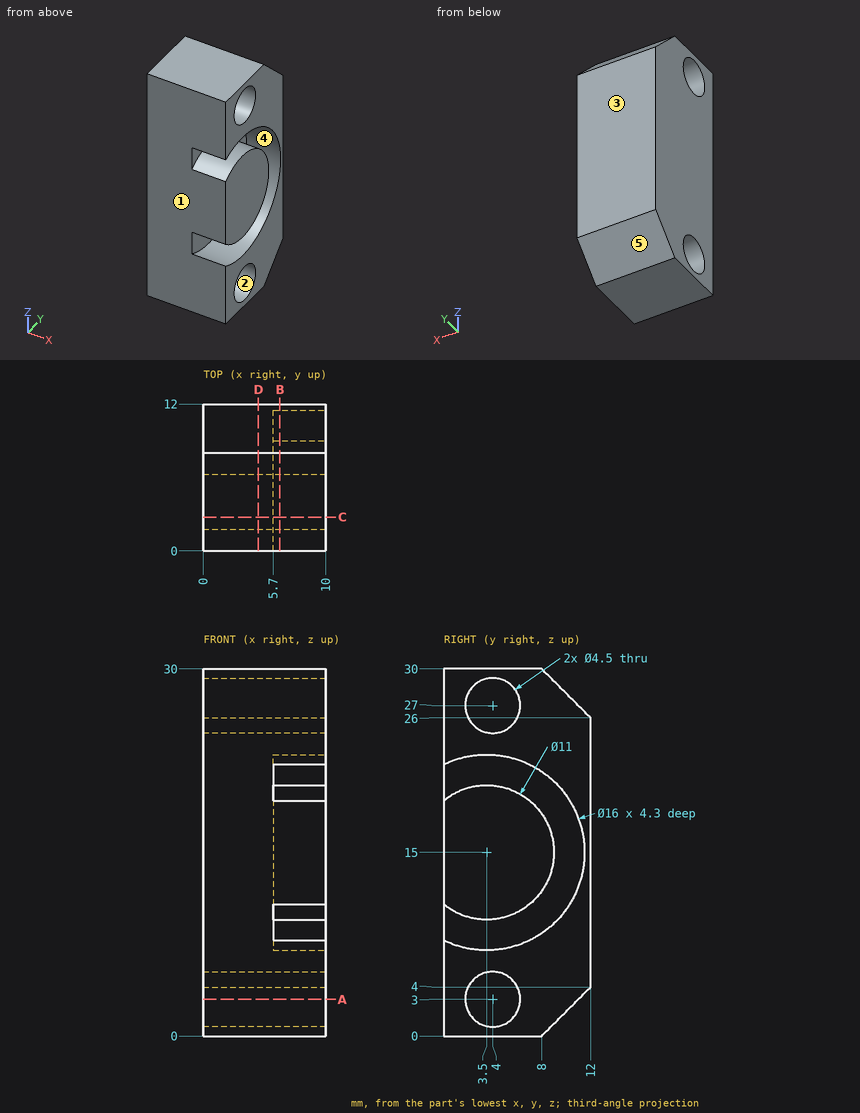
Study the drawing (mm; zero at the part's minimum x, y, z) and answer. A direction names the side the tool comes from. Coordinates: 2 decimals unless noted, no trailing zeros. Loops run counter-clockwise (first coordinate to the right, second up) from the corner with the lowest first, then second, coordinate; pieces in that order, holes last. Notation, with made-up numbers: M 17,87 L 69,87 A24 cw 69,116 Z; hole C -14,70.25 d9. An arc over 180 degrees is marked long. Answer as a JSON object with one key per item and string values. Group by question number.
Item 1: Which of the six approach directions +Z, -Z, +X, -X, +Y, -Y give full straight-line access (tool end or side, diameter ignored) to the marked faces 4 and 5?
Item 2: Determine the mould class of the marked faces 1, 2 and 3 for opening direction Y: +Y half, -Y half, draft (parallel to the pull), parting line (faces both ways), or undercut.
Item 3: Section C-C (y = 2.75) is taken. Write down the section's boundary in (x, z).
Item 4: Section D-D (x = 4.5) is taken. Write down the section's boundary in (y, z).
Item 5: Section B-B (x = 6.25) is taken. Write down the section's boundary in (y, z), and give its area (3 significant figures).
Item 6: Consider L1, parallel to Z at x = 6.25, y = 1.25; L2, parallel to Y at x = 7, z = 15; L3, parallel to Z at x = 8.4, y = 3.5. Determine where each line is inside the solid, lowest interval first.
Item 7: Section A-A (z = 3) is taken. Write down the section's boundary in (x, y).
Item 8: This flat-tipped pin is pushed along its axis until it touches: P1, Ø2.5, axis at y = 4, z = 3, coming from the +X side. Where does it stop, or does it pass through?
Solved:
{
 "1": {"face 4": "+X", "face 5": "-Z, +X, -X, +Y"},
 "2": {"face 1": "-Y half", "face 2": "undercut", "face 3": "+Y half"},
 "3": {"outline": "M 0,0 L 10,0 L 10,1.13 L 0,1.13 Z; M 0,4.87 L 10,4.87 L 10,7.04 L 5.7,7.04 L 5.7,9.55 L 10,9.55 L 10,20.45 L 5.7,20.45 L 5.7,22.96 L 10,22.96 L 10,25.13 L 0,25.13 Z; M 0,28.87 L 10,28.87 L 10,30 L 0,30 Z"},
 "4": {"outline": "M 0,0 L 8,0 L 12,4 L 12,26 L 8,30 L 0,30 Z; hole C 4,3 d4.5; hole C 4,27 d4.5"},
 "5": {"outline": "M 0,0 L 8,0 L 12,4 L 12,26 L 8,30 L 0,30 L 0,22.19 A8 cw long 0,7.81 Z; M 0,10.76 A5.5 ccw long 0,19.24 Z; hole C 4,3 d4.5; hole C 4,27 d4.5", "area": "241 mm2"},
 "6": {"L1": "z = 0 to 7.32, 9.98 to 20.02, 22.68 to 30", "L2": "y = 0 to 9, 11.5 to 12", "L3": "z = 0 to 0.81, 5.19 to 7, 9.5 to 20.5, 23 to 24.81, 29.19 to 30"},
 "7": {"outline": "M 0,0 L 10,0 L 10,1.75 L 0,1.75 Z; M 0,6.25 L 10,6.25 L 10,11 L 0,11 Z"},
 "8": {"P1": "passes through"}
}
